Source: three-view drawing plus pictorial views. Frame: mm from the lowest corner of the part. Coordinates: 2 decimals unless noted, no trailing zeros. Loops run counter-clockwise (first coordinate to the right, second up) from the corner with the lowest first, then second, coordinate; pieces in that order, holes last. Notation, with made-up numbers: M -37.75,13.25 L -0.75,13.25 A23 ccw -0.75,24.25 Z; hole C -2,48 d8. An arc over 180 degrees is marked long. Use a Markdown table: item, result. Add a question column.
1. Section B-B on y = 31.75. Output: boundary loops of the cut face in (x, z), then the cut area to 3 significant figures.
2. Section D-D on y = 52.5. Output: boundary loops of the cut face in (x, z).
3. Pin query (flat end, axial travel): pin 1 (1.4 mm diameter, centred on y = 10.5, z = 3.5, fed in from +X); pin 2 (1.4 mm diameter, centred on x = 73.5, z = 2.5, fed in from -Y) (1 decimal); pin 3 (2.5 mm diameter, centred on x = 2, z = 2.5, fed in from +Y) (1 decimal). Return the tip coordinate at first contact, or that it passes through.
4. Line query: L1, parallel to Y at x = 38.1, z = 2.75; L2, parallel to Y at x = 73, z = 1 (1 decimal); L3, parallel to X at y = 9, z = 4.45. Output: solid intervals per line, ascending. Write a range as [from, to].
5. Section A-A on x = 38.1. Output: boundary loops of the cut face in (y, z).
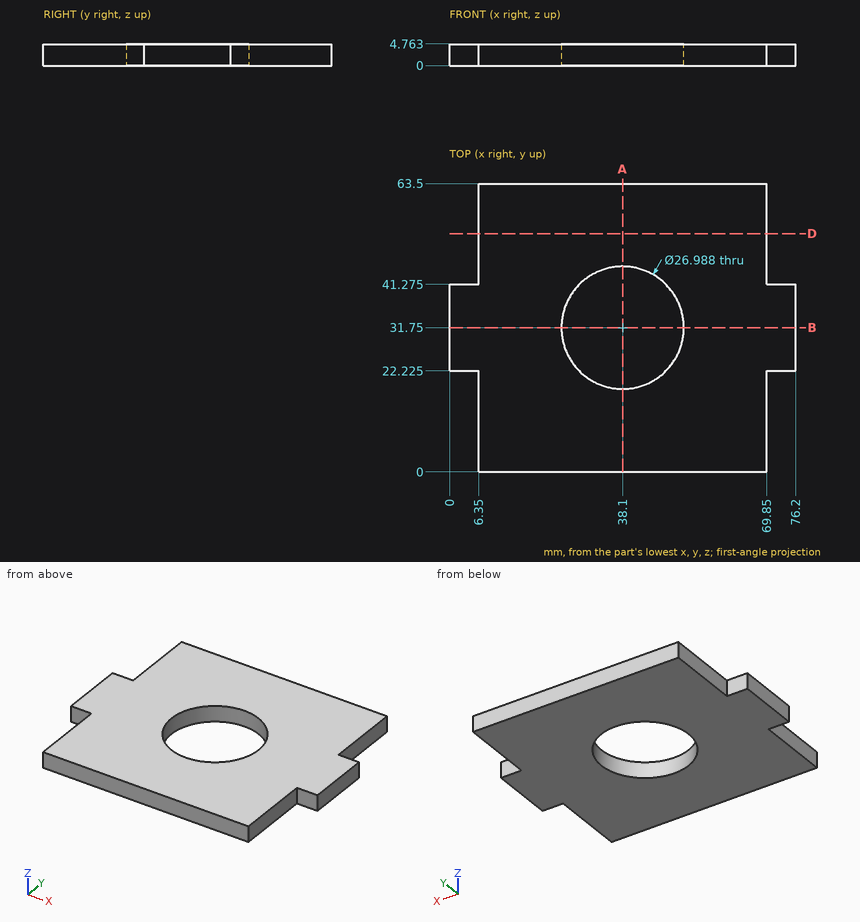
Answers below:
| question | item | result |
|---|---|---|
| 1 | outline | M 0,0 L 24.61,0 L 24.61,4.76 L 0,4.76 Z; M 51.59,0 L 76.2,0 L 76.2,4.76 L 51.59,4.76 Z |
| 1 | area | 234 mm² |
| 2 | outline | M 6.35,0 L 69.85,0 L 69.85,4.76 L 6.35,4.76 Z |
| 3 | pin 1 | stops at x = 69.85 |
| 3 | pin 2 | stops at y = 22.2 |
| 3 | pin 3 | stops at y = 41.3 |
| 4 | L1 | y = [0, 18.26], [45.24, 63.5] |
| 4 | L2 | y = [22.2, 41.3] |
| 4 | L3 | x = [6.35, 69.85] |
| 5 | outline | M 0,0 L 18.26,0 L 18.26,4.76 L 0,4.76 Z; M 45.24,0 L 63.5,0 L 63.5,4.76 L 45.24,4.76 Z |
